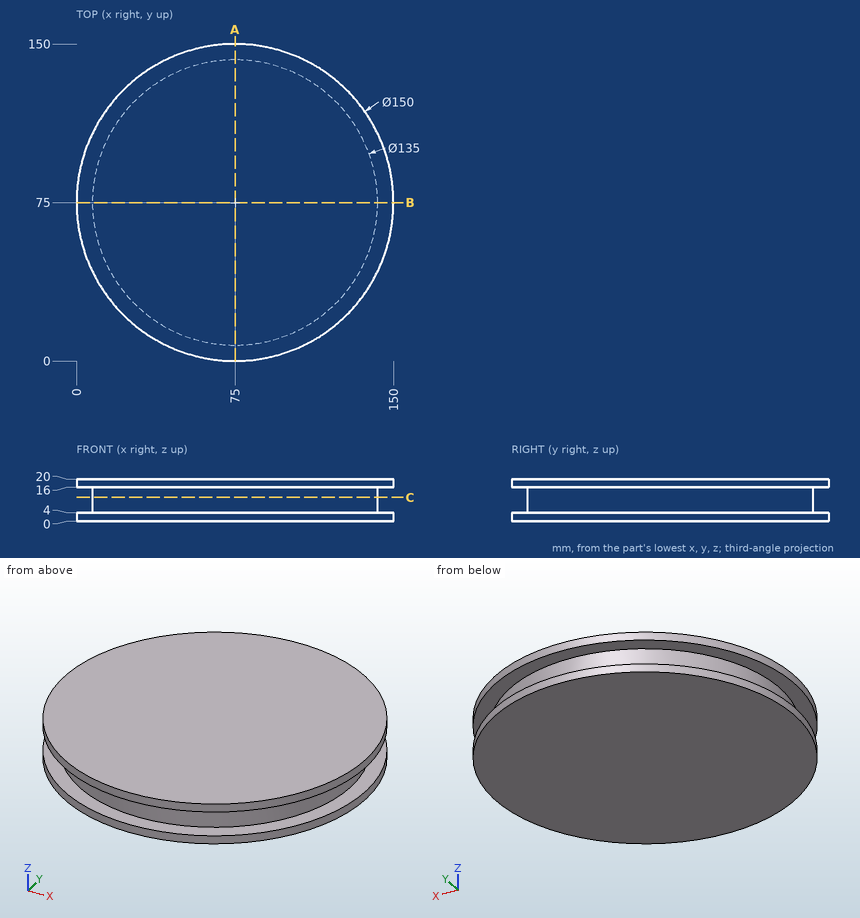
Could you check a few things on this drawing? It's one solid part, dimensions in mm from its lowest x, y, z. Coordinates: 2 decimals unless noted, no trailing zeros. Order: outer loops, then holes, each group sorted by start corner. A loop starts at its lowest first (then second) coordinate and runs counter-clockwise, first axis right, second up. Notation, with made-up numbers: M 58.25,13.25 L 116.25,13.25 A26 ccw 116.25,28.25 Z; hole C 30,69.25 d3. An arc over 180 degrees is marked long. Answer as a JSON object with one key per item and string values. Group by question number.
(1) Suppose I cut it at C-C, the plane z = 11.25. Please give me the cut outline in (x, y), then the cut area to 3 significant figures.
(2) For pin 1 (2 mm diameter, centred on x = 102, z = 13.5, fed in from -Y); pin 2 (8 mm diameter, centred on x = 60.5, z = 2.5, fed in from +Y); pin 3 (1 mm diameter, centred on y = 52, z = 15, fed in from +X), each with a flat end and sliding along its axis, tell me the tip position at first contact or that it passes through.
(3) I need wall thicknesses on probe 1 along Z at (x, y) = (50, 8.5); probe 2 along Y at (x, z) = (121.5, 15); probe 3 along X at (y, z) = (39, 5.25). Which ranges of each line are inside material? Lowest first, please.
(4) Suppose I cut it at A-A, the plane x = 75. Please give me the cut outline in (y, z), then the cut area to 3 significant figures.
Values found:
{
 "1": {"outline": "C 75,75 d135", "area": "14,300 mm^2"},
 "2": {"pin 1": "stops at y = 12.71", "pin 2": "stops at y = 149.26", "pin 3": "stops at x = 138.64"},
 "3": {"probe 1": "z = 0 to 4, 16 to 20", "probe 2": "y = 26.07 to 123.93", "probe 3": "x = 17.9 to 132.1"},
 "4": {"outline": "M 0,0 L 150,0 L 150,4 L 142.5,4 L 142.5,16 L 150,16 L 150,20 L 0,20 L 0,16 L 7.5,16 L 7.5,4 L 0,4 Z", "area": "2,820 mm^2"}
}
